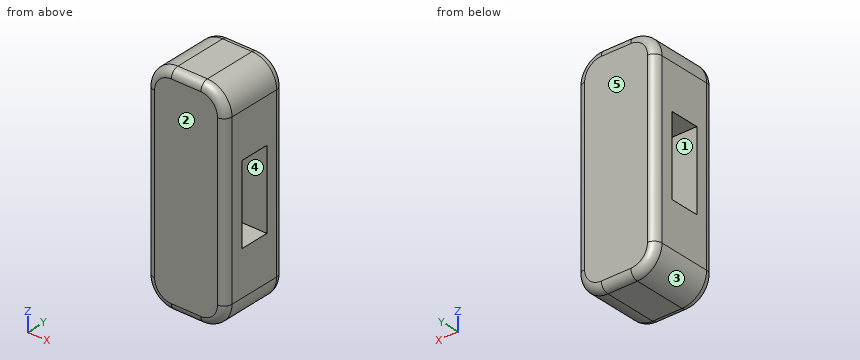
from build123d import *

# Parameters (mm, degrees)
F1_DEPTH = 44.45
F2_R     = 5.08
F3_W     = 19.267222
F3_H     = 50.8
F4_DEPTH = 50.801


with BuildPart() as f1:
    # F0 (on Front) → F1 (new body)
    with BuildSketch(Plane.XZ):
        with BuildLine():
            ThreePointArc((-25.4, -53.975), (-20.75032, -65.20032), (-9.525, -69.85))
            Line((-9.525, -69.85), (9.525, -69.85))
            ThreePointArc((9.525, -69.85), (20.75032, -65.20032), (25.4, -53.975))
            Line((25.4, -53.975), (25.4, 53.975))
            ThreePointArc((25.4, 53.975), (20.75032, 65.20032), (9.525, 69.85))
            Line((9.525, 69.85), (-9.525, 69.85))
            ThreePointArc((-9.525, 69.85), (-20.75032, 65.20032), (-25.4, 53.975))
            Line((-25.4, 53.975), (-25.4, -53.975))
        make_face()
    extrude(amount=F1_DEPTH)

    # F2
    f2_edges = [f1.edges().sort_by_distance(p)[0] for p in [
        (0, -44.45, 69.85),
        (-20.75032, -44.45, -65.20032),
        (0, -44.45, -69.85),
        (20.75032, -44.45, -65.20032),
        (25.4, -44.45, 0),
        (20.75032, -44.45, 65.20032),
        (-20.75032, -44.45, 65.20032),
        (-25.4, -44.45, 0),
        (0, 0, 69.85),
        (25.4, 0, 0),
    ]]
    fillet(f2_edges, radius=F2_R)

    # F3 (on face) → F4 (cut, through all)
    with BuildSketch(Plane.YZ.offset(25.4)):
        with Locations((-22.225, 0)):
            Rectangle(F3_W, F3_H)
    extrude(amount=-F4_DEPTH, mode=Mode.SUBTRACT)


solid = f1.part
Geometry check sheet. Reference: the model listing, model coordinates, mm. Face numbers are marked on the shaded views. A direction names the side the tool comes from. Give positions to 0.01 mm unless a question says otherwise; leave off trailing zeros. Write each loop counter-clockwise with the first axis right and the second up, starting at its lowest first coordinate (ties: lowest second). Pieces come first, ordered by that corner, then holes. Notation, with made-up numbers: M 2.25,9.25 L 15.25,9.25 A24 cw 15.25,28.25 Z; hole C -18.5,67 d2. An arc over 180 degrees is marked long. Answer as CSV lines item,"result". Start each with the question number.
Q1. Release check for a two-part mould opening along Z. For the marked faces 1, 2 and 3 record: pulls with the +Z half, pulls with the -Z half, needs draft (parallel to the pull), parting line crosses it, or undercut.
Q2. Section check D-D, the plane y = -3. Record the cut outline in (x, z) (3 decimals).
Q3. Section check B-B, the plane y = -29. Record the cut outline in (x, z) (3 decimals).
Q4. Section check C-C, the plane x = -1. Record the cut outline in (y, z), then the cut area to 3 significant figures.
Q5. Tool access check on the marked faces 4 and 5. Record the directions out of +Z, -Z, +X, -X, +Y, -Y that give a thin tool (end or side, any length) a straight path to the whole face; none if there is none.
Q6. Material ranges on L1, parallel to Y at x = -3, z = 4; L2, parallel to Z at x = -9.5, y = -14; L3, parallel to Z at x = -15, y = -18, recorded low to high.
Q7. Go/stop test with a flat-tipped pin: pin 1 (8 mm diameter, centred on x = 17.5, y = -29.5, fed in from -Z). Record where the tip stops, or that it passes through.
Q8. Section check A-A, the plane z = -17. Record the cut outline in (x, y), then the cut area to 3 significant figures.
Geometry says:
1,face 1,"undercut"
1,face 2,"needs draft"
1,face 3,"pulls with the -Z half"
2,outline,"M -24.955,-53.975 A15.43 ccw -9.525,-69.405 L 9.525,-69.405 A15.43 ccw 24.955,-53.975 L 24.955,53.975 A15.43 ccw 9.525,69.405 L -9.525,69.405 A15.43 ccw -24.955,53.975 Z"
3,outline,"M -25.4,-53.975 A15.875 ccw -9.525,-69.85 L 9.525,-69.85 A15.875 ccw 25.4,-53.975 L 25.4,-25.4 L -25.4,-25.4 Z; M -25.4,25.4 L 25.4,25.4 L 25.4,53.975 A15.875 ccw 9.525,69.85 L -9.525,69.85 A15.875 ccw -25.4,53.975 Z"
4,outline,"M -44.45,-64.77 A5.08 ccw -39.37,-69.85 L -5.08,-69.85 A5.08 ccw 0,-64.77 L 0,64.77 A5.08 ccw -5.08,69.85 L -39.37,69.85 A5.08 ccw -44.45,64.77 Z; hole M -31.86,-25.4 L -12.59,-25.4 L -12.59,25.4 L -31.86,25.4 Z"
4,area,"5,210 mm^2"
5,face 4,"+X, -X"
5,face 5,"+Z, -Z, +X, -X, +Y"
6,L1,"-44.45 to -31.86, -12.59 to 0"
6,L2,"-69.85 to -25.4, 25.4 to 69.85"
6,L3,"-68.88 to -25.4, 25.4 to 68.88"
7,pin 1,"z = -69.34"
8,outline,"M -25.4,-39.37 A5.08 ccw -20.32,-44.45 L 20.32,-44.45 A5.08 ccw 25.4,-39.37 L 25.4,-31.86 L -25.4,-31.86 Z; M -25.4,-12.59 L 25.4,-12.59 L 25.4,-5.08 A5.08 ccw 20.32,0 L -20.32,0 A5.08 ccw -25.4,-5.08 Z"
8,area,"1,260 mm^2"
